Input: part model. Units: mm. Frame: model coordinates. Face numbers are marked on the shaded views. A direction names the side the tool comes from. Round coordinates to 2 decimals unless told otherwise and drop trailing zeros. Order: outer loops, then holes, each group sorted by start corner. A loop starts at its lowest first (then second) coordinate and runs counter-clockwise, first axis right, second up.
Item 1: Reachability of the marked faces 4, 5 and 6 from +Z, -Z, +X, -X, +Y, -Y: full face, straight path, thin tool, end or side. Return the list, or none.
Item 2: Mould query, pull axis X, two halves, no side actions, for the marked faces 1, 2 and 3. Classes: released by +X, released by -X, zero draft, split by the parting line, or undercut.
Item 3: Cut plane B-B on y = 13.75. Output: boundary loops of the cut face in (x, z), then the cut area to 3 significant figures.
Item 4: Line query: L1, parallel to X at y = 2.25, z = 16.5; L2, parallel to Y at x = -24, z = 6.75; L3, parallel to Y at x = -16, z = 3.5. Output: solid intervals per line, ascending.
Item 5: Cut plane A-A on z = 2. Output: boundary loops of the cut face in (x, y), then the cut area to 3 significant figures.
Item 6: Cut plane C-C on x = -15.5. Output: boundary loops of the cut face in (y, z), then the cut area to 3 significant figures.
Item 7: First-contact query: pin 1 (4 mm diameter, centred on y = 1, z = 15, fed in from -X); pin 2 (1.5 mm diameter, centred on y = 15, z = 17.5, fed in from -X); pin 3 (1.2 mm diameter, centred on x = -24, y = 11.5, fed in from -Z). Flat tips, straight axial feed; report the tip coordinate or a pass-through.
Item 8: Cut plane D-D on z = 11.5. Output: boundary loops of the cut face in (x, y), then the cut area to 3 significant figures.
```python
from build123d import *

# Parameters (mm, degrees)
EXTRUDE_1_DEPTH     = 21
EXTRUDE_2_DEPTH     = 9.3
CUT_EXTRUDE_1_DEPTH = 0.1
FILLET_1_R          = 3
FILLET_2_R          = 1


with BuildPart() as part:
    # 草图1 → 凸台-拉伸1 (new body)
    with BuildSketch(Plane.XY):
        Polygon((0, 17.4), (0, 0), (-11.3, 0), (-11.3, 6.8), (-21, 6.8), (-21, 17.4), align=None)
    extrude(amount=EXTRUDE_1_DEPTH)

    # 草图2 → 凸台-拉伸2 (add)
    with BuildSketch(Plane.ZY.offset(21)):
        Polygon((5.5, 14.35), (3.5, 12.35), (3.5, 9.85), (17.5, 9.85), (17.5, 12.35), (15.5, 14.35), align=None)
    extrude(amount=EXTRUDE_2_DEPTH)

    # 草图3 → 切除-拉伸1 (cut)
    with BuildSketch(Plane.XZ):
        Polygon((-7.9, 3.5), (-5.4, 3.5), (-3.4, 5.5), (-3.4, 15.5), (-5.4, 17.5), (-7.9, 17.5), align=None)
    extrude(amount=-CUT_EXTRUDE_1_DEPTH, mode=Mode.SUBTRACT)

    # 圆角1
    fillet_1_edges = [part.edges().sort_by_distance(p)[0] for p in [
        (0, 17.4, 10.5),
        (-11.3, 6.8, 10.5),
    ]]
    fillet(fillet_1_edges, radius=FILLET_1_R)

    # 圆角2
    fillet_2_edges = [part.edges().sort_by_distance(p)[0] for p in [
        (-5.65, 0, 21),
        (0, 7.2, 21),
        (-21, 12.1, 21),
        (-11.3, 1.9, 0),
        (-11.3, 1.9, 21),
        (-12, 17.4, 0),
        (-12, 17.4, 21),
        (-0.878679656, 16.521320344, 0),
        (-0.878679656, 16.521320344, 21),
        (-12.178679656, 5.921320344, 0),
        (-12.178679656, 5.921320344, 21),
        (0, 7.2, 0),
        (-5.65, 0, 0),
        (-17.65, 6.8, 21),
        (-17.65, 6.8, 0),
        (-21, 12.1, 0),
    ]]
    fillet(fillet_2_edges, radius=FILLET_2_R)


solid = part.part
```
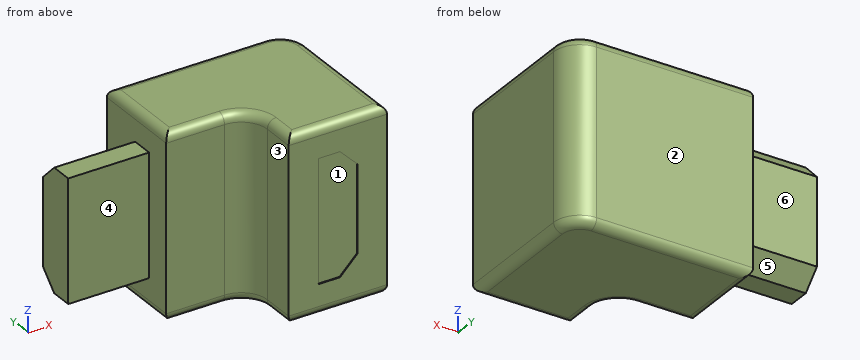
From the geometry:
1. face 4: +Z, -Z, -X, -Y
1. face 5: -Z, -X, +Y
1. face 6: +Z, -Z, -X, +Y
2. face 1: undercut
2. face 2: zero draft
2. face 3: released by -X
3. outline: (-30.3, 4.9) - (-21, 4.9) - (-21, 1) arc R1 ccw to (-20, 0) - (-1, 0) arc R1 ccw to (0, 1) - (0, 20) arc R1 ccw to (-1, 21) - (-20, 21) arc R1 ccw to (-21, 20) - (-21, 16.1) - (-30.3, 16.1) - close
3. area: 544 mm2
4. L1: x = -11.3 to 0
4. L2: y = 9.85 to 14.35
4. L3: y = 6.8 to 17.4
5. outline: (-21, 6.8) - (-14.3, 6.8) arc R3 cw to (-11.3, 3.8) - (-11.3, 0) - (0, 0) - (0, 14.4) arc R3 ccw to (-3, 17.4) - (-21, 17.4) - close
5. area: 299 mm2
6. outline: (6.8, 1) arc R1 ccw to (7.8, 0) - (16.4, 0) arc R1 ccw to (17.4, 1) - (17.4, 20) arc R1 ccw to (16.4, 21) - (7.8, 21) arc R1 ccw to (6.8, 20) - close
6. area: 222 mm2
7. pin 1: stops at x = -11.3
7. pin 2: stops at x = -21
7. pin 3: stops at z = 3.5
8. outline: (-30.3, 9.85) - (-21, 9.85) - (-21, 6.8) - (-14.3, 6.8) arc R3 cw to (-11.3, 3.8) - (-11.3, 0) - (-7.9, 0) - (-7.9, 0.1) - (-3.4, 0.1) - (-3.4, 0) - (0, 0) - (0, 14.4) arc R3 ccw to (-3, 17.4) - (-21, 17.4) - (-21, 14.35) - (-30.3, 14.35) - close
8. area: 341 mm2
